Answer from the drawing. Dimensions are ordinates in mm from the lowest x, y and z of the part. A direction names the side the tool comes from. Round coordinates to 2 decimals unless told otherwise and drop trailing zeros. Order: outer loops, then holes, each group sorted by start corner. A loop starts at its lowest first (then second) coordinate and runs counter-clockwise, first axis right, second up. Notation, with made-up numbers: (3, 10.5) -> (22, 10.5) arc R21 ccw to (22, 21.5) -> close; hole circle Ø2 at (-38, -30). An arc over 180 degrees is marked (long way). Use a Markdown table: item, result. Add a question column.
Item 1: A cutting plane is placed at A-A, the plane x = 10. Determine the outline of the cut face in (y, z), plus the area to 3 significant figures.
Item 2: A tool of negligible diameter and unlimited length cuts with its end or side. For the marked faces 4 and 5, from which of +Z, -Z, +X, -X, +Y, -Y can it reach the whole face along a straight path? Write none if from no direction.
Item 3: A cutting plane is placed at C-C, the plane y = 7. Determine the outline of the cut face in (x, z), plus the area to 3 significant figures.
Item 4: Find the intervals of material crossed by L1, parallel to Y at x = 15.25, z = 0.8 (1 decimal); L2, parallel to X at y = 15.75, z = 0.4; L3, parallel to X at y = 5.25, z = 1.8, in increasing order. Write a range as [from, to].
Item 5: A cutting plane is placed at D-D, the plane z = 0.55. Give the number of separate pieces and of enclosed holes in the cut face, plus the area to 3 significant figures.
Item 6: Flat-ended cylindrical pins translate along their axes: P1, Ø1.6, axis at x = 10, y = 3, coming from the +Z side; P2, Ø6, axis at x = 8.5, y = 10, coming from the +Z side. Find the tip coordinate at first contact, or state that the pin passes through.
Item 7: For a pull along Y with two mould halves and no side action, classify the marked faces 1, 2 and 3 as +Y half, -Y half, draft (parallel to the pull), parting line (faces both ways), or undercut.
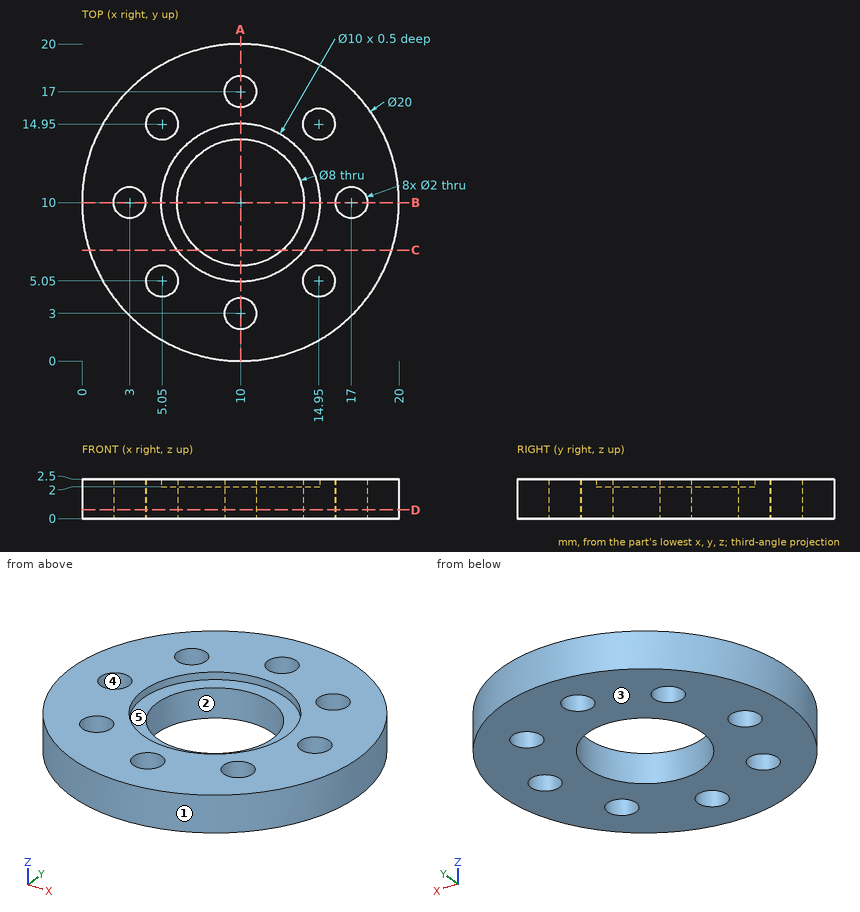
Reported:
| question | item | result |
|---|---|---|
| 1 | outline | (0, 0) -> (2, 0) -> (2, 2.5) -> (0, 2.5) -> close; (4, 0) -> (6, 0) -> (6, 2) -> (5, 2) -> (5, 2.5) -> (4, 2.5) -> close; (14, 0) -> (16, 0) -> (16, 2.5) -> (15, 2.5) -> (15, 2) -> (14, 2) -> close; (18, 0) -> (20, 0) -> (20, 2.5) -> (18, 2.5) -> close |
| 1 | area | 19.0 mm² |
| 2 | face 4 | +Z, -Z |
| 2 | face 5 | +Z |
| 3 | outline | (0.46, 0) -> (7.35, 0) -> (7.35, 2) -> (6, 2) -> (6, 2.5) -> (0.46, 2.5) -> close; (12.65, 0) -> (19.54, 0) -> (19.54, 2.5) -> (14, 2.5) -> (14, 2) -> (12.65, 2) -> close |
| 3 | area | 33.1 mm² |
| 4 | L1 | [1.5, 4.1], [6, 14], [15.9, 18.5] |
| 4 | L2 | [1.82, 4.45], [5.65, 14.35], [15.55, 18.18] |
| 4 | L3 | [1.2, 4.07], [6.03, 13.97], [15.93, 18.8] |
| 5 | separate pieces | 1 |
| 5 | enclosed holes | 9 |
| 5 | area | 239 mm² |
| 6 | P1 | through |
| 6 | P2 | z = 2 |
| 7 | face 1 | parting line |
| 7 | face 2 | undercut |
| 7 | face 3 | draft |
